```python
from build123d import *

# Parameters (mm, degrees)
F0_W     = 304.8
F0_H     = 90.5500094
F0_W_2   = 11.5876832
F0_H_2   = 24
F1_DEPTH = 3.175
F2_R     = 2.15265
F3_DEPTH = 3.175
F4_W     = 9.525
F4_H     = 9.525
F5_DEPTH = 3.175


with BuildPart() as f1:
    # F0 (on Top) → F1 (new body)
    with BuildSketch(Plane.XY):
        with Locations((152.4, -45.2750047)):
            Rectangle(F0_W, F0_H)
        with Locations((50.8, -75.3750094)):
            Rectangle(F0_W_2, F0_H_2, mode=Mode.SUBTRACT)
        with Locations((254, -75.3750094)):
            Rectangle(F0_W_2, F0_H_2, mode=Mode.SUBTRACT)
        with Locations((50.8, -15.175)):
            Rectangle(F0_W_2, F0_H_2, mode=Mode.SUBTRACT)
        with Locations((254, -15.175)):
            Rectangle(F0_W_2, F0_H_2, mode=Mode.SUBTRACT)
    extrude(amount=F1_DEPTH)

    # F2 (on face) → F3 (cut, through all)
    with BuildSketch(Plane.XY.offset(3.175)):
        with Locations((4.7625, -14.2875)):
            Circle(F2_R)
        with Locations((4.7625, -76.2625094)):
            Circle(F2_R)
        with Locations((300.0375, -76.2625094)):
            Circle(F2_R)
        with Locations((300.0375, -14.2875)):
            Circle(F2_R)
    extrude(amount=-F3_DEPTH, mode=Mode.SUBTRACT)

    # F4 (on face) → F5 (cut, through all)
    with BuildSketch(Plane.XY.offset(3.175)):
        with Locations((300.0375, -4.7625)):
            Rectangle(F4_W, F4_H)
        with Locations((300.0375, -85.7875094)):
            Rectangle(F4_W, F4_H)
        with Locations((4.7625, -85.7875094)):
            Rectangle(F4_W, F4_H)
        with Locations((4.7625, -4.7625)):
            Rectangle(F4_W, F4_H)
    extrude(amount=-F5_DEPTH, mode=Mode.SUBTRACT)


solid = f1.part
```
Geometry check sheet. Reference: the model listing, model coordinates, mm. Round coordinates to 2 decimals unless told otherwise and drop trailing zeros. Order: outer loops, then holes, each group sorted by start corner. A loop starts at its lowest first (then second) coordinate and runs counter-clockwise, first axis right, second up. Notation, with made-up numbers: (75, 28) -> (113, 28) arc R21 cw to (113, 40) -> close; hole circle Ø10 at (72, 84). An arc over 180 degrees is marked (long way). Return JSON: item names as keys, results as strings. Group by question number.
Q1. Gauge pin test, flat ends, axial feed: pin 1 (6 mm diameter, centred on x = 112, y = -12.5, fed in from -Z); pin 2 (1.6 mm diameter, centred on x = 301.5, z = 2, fed in from +Y) (3 decimals); pin 3 (1 mm diameter, centred on y = -5, z = 2, fed in from +X) (3 decimals). Record the tip position at first contact, or that the pin passes through.
Q2. Material ranges on probe 1 along X at (y, z) = (-21.5, 2.1); probe 2 along Y at (x, z) = (252, 1.5) (3 decimals); probe 3 along X at (y, z) = (-14, 2.5), recorded low to high. Write a range as from..to.
Q3. Section check B-B, the plane z = 0.65. Count the separate pieces of the cut face and the enclosed holes in it, plus the area to 3 significant figures.
Q4. Section check A-A, the plane y = -66. Record the boundary of the cut face in (x, z) (3 decimals).
Numbers:
{
 "1": {"pin 1": "z = 0", "pin 2": "y = -9.525", "pin 3": "x = 295.275"},
 "2": {"probe 1": "0..45.01, 56.59..248.21, 259.79..304.8", "probe 2": "-90.55..-87.375, -63.375..-27.175, -3.175..0", "probe 3": "0..2.63, 6.9..45.01, 56.59..248.21, 259.79..297.9, 302.17..304.8"},
 "3": {"separate pieces": "1", "enclosed holes": "8", "area": "26,100 mm^2"},
 "4": {"outline": "(0, 0) -> (45.006, 0) -> (45.006, 3.175) -> (0, 3.175) -> close; (56.594, 0) -> (248.206, 0) -> (248.206, 3.175) -> (56.594, 3.175) -> close; (259.794, 0) -> (304.8, 0) -> (304.8, 3.175) -> (259.794, 3.175) -> close"}
}
